Input: part model. Units: mm. Frame: model coordinates. A direction names the side the tool comes from. Give positions to 0.01 mm unless a question says otherwise; leave off trailing zeros. Loops run counter-clockwise (first coordinate to the right, second up) from the corner with the lowest first, then second, coordinate; pieces in that order, holes last. Notation, with made-up numbers: (-17, 84.25) -> (23, 84.25) arc R17 cw to (23, 89.25) -> close; hole circle Ø3 at (-32.5, 34.25). An arc over 180 degrees is marked (long way). Use CSV: the item, a comma, the result in double quotes.
```python
from build123d import *

# Parameters (mm, degrees)
SKETCH1_W                       = 126
SKETCH1_H                       = 106
BOSS_EXTRUDE1_DEPTH             = 5
SKETCH3_W                       = 126
SKETCH3_H                       = 106
SKETCH3_W_2                     = 122
SKETCH3_H_2                     = 102
BOSS_EXTRUDE3_DEPTH             = 5
BOSS_EXTRUDE5_DEPTH             = 4
FILLET1_R                       = 3
F_4_0MM_DOWEL_HOLE1_D           = 4
F_4_0MM_DOWEL_HOLE1_CSINK_D     = 8
F_4_0MM_DOWEL_HOLE1_CSINK_ANGLE = 90
SKETCH17_R                      = 1.15
BOSS_EXTRUDE6_DEPTH             = 10
SKETCH18_W                      = 3
SKETCH18_H                      = 3
BOSS_EXTRUDE7_DEPTH             = 4
SKETCH4_R                       = 3.75
BOSS_EXTRUDE8_DEPTH             = 4
F_2_5MM_DOWEL_HOLE1_D           = 2.5


with BuildPart() as part:
    # Sketch1 → Boss-Extrude1 (new body)
    with BuildSketch(Plane(origin=(0, 0, 0), x_dir=(1, 0, 0), z_dir=(0, 1, 0))):
        Rectangle(SKETCH1_W, SKETCH1_H)
    extrude(amount=BOSS_EXTRUDE1_DEPTH)

    # Sketch3 → Boss-Extrude3 (add)
    with BuildSketch(Plane(origin=(0, 5, 0), x_dir=(1, 0, 0), z_dir=(0, 1, 0))):
        Rectangle(SKETCH3_W, SKETCH3_H)
        Rectangle(SKETCH3_W_2, SKETCH3_H_2, mode=Mode.SUBTRACT)
    extrude(amount=BOSS_EXTRUDE3_DEPTH)

    # Sketch7 → Boss-Extrude5 (add)
    with BuildSketch(Plane(origin=(0, 0, 0), x_dir=(1, 0, 0), z_dir=(0, 1, 0))):
        with BuildLine():
            Line((-63, 43), (-73, 43))
            ThreePointArc((-73, 43), (-78, 38), (-73, 33))
            Line((-73, 33), (-63, 33))
            Line((-63, 33), (-63, 43))
        make_face()
        with BuildLine():
            Line((63, -33), (73, -33))
            ThreePointArc((73, -33), (78, -38), (73, -43))
            Line((73, -43), (63, -43))
            Line((63, -43), (63, -33))
        make_face()
    extrude(amount=BOSS_EXTRUDE5_DEPTH)

    # Fillet1
    fillet1_edges = [part.edges().sort_by_distance(p)[0] for p in [
        (-63, 2, -33),
        (-63, 2, -43),
        (63, 2, 33),
        (63, 2, 43),
    ]]
    fillet(fillet1_edges, radius=FILLET1_R)

    # Ø4.0mm Dowel Hole1 (through all)
    with Locations(Plane(origin=(0, 4, 0), x_dir=(1, 0, 0), z_dir=(0, 1, 0))):
        with Locations((-73, 38), (73, -38)):
            CounterSinkHole(F_4_0MM_DOWEL_HOLE1_D / 2, F_4_0MM_DOWEL_HOLE1_CSINK_D / 2, counter_sink_angle=F_4_0MM_DOWEL_HOLE1_CSINK_ANGLE)

    # Sketch17 → Boss-Extrude6 (add)
    with BuildSketch(Plane(origin=(0, 5, 0), x_dir=(1, 0, 0), z_dir=(0, 1, 0))):
        with Locations(Location((-55.626, -15.47, 0), (0, 0, 90))):
            Circle(SKETCH17_R)
        with Locations(Location((55.626, -15.47, 0), (0, 0, 90))):
            Circle(SKETCH17_R)
    extrude(amount=BOSS_EXTRUDE6_DEPTH)

    # Sketch18 → Boss-Extrude7 (add)
    with BuildSketch(Plane(origin=(0, 5, 0), x_dir=(1, 0, 0), z_dir=(0, 1, 0))):
        with Locations((-59.5, 49.5)):
            Rectangle(SKETCH18_W, SKETCH18_H)
        with Locations((59.5, 49.5)):
            Rectangle(SKETCH18_W, SKETCH18_H)
        with Locations((-59.5, -49.5)):
            Rectangle(SKETCH18_W, SKETCH18_H)
        with Locations((59.5, -49.5)):
            Rectangle(SKETCH18_W, SKETCH18_H)
    extrude(amount=BOSS_EXTRUDE7_DEPTH)

    # Sketch4 → Boss-Extrude8 (add)
    with BuildSketch(Plane(origin=(0, 5, 0), x_dir=(1, 0, 0), z_dir=(0, 1, 0))):
        with Locations(Location((0, 13.486, 0), (0, 0, 90))):
            Circle(SKETCH4_R)
    extrude(amount=BOSS_EXTRUDE8_DEPTH)

    # Ø2.5mm Dowel Hole1 (through all)
    with Locations(Plane(origin=(0, 9, 0), x_dir=(1, 0, 0), z_dir=(0, 1, 0))):
        with Locations((0, 13.486)):
            Hole(F_2_5MM_DOWEL_HOLE1_D / 2)


solid = part.part
```
1) Ray query, line 1 (Z direction, x = -73, y = 0.7); line 2 (Z direction, x = 73, y = 1.4); line 3 (X direction, y = 0.65, z = -38). Return the intervals inside material, ascending.
From the geometry:
line 1,"z = -43 to -40, -36 to -33"
line 2,"z = 33 to 36, 40 to 43"
line 3,"x = -78 to -75, -71 to 63"
2) Section query D-D (z = -28). Return loops of the section in (x, y).
From the geometry:
outline,"(-63, 0) -> (63, 0) -> (63, 10) -> (61, 10) -> (61, 5) -> (-61, 5) -> (-61, 10) -> (-63, 10) -> close"
3) Reachability of faces 1 (the cylindrical face through (-63.86, 2.03, -43.9)), 2 (the flat face through (-60, 7, 48)) from +Z, -Z, +X, -X, +Y, -Y: full face, straight path, thin tool, end or side. Return the list, or none.
From the geometry:
face 1,"-Z, -X, +Y, -Y"
face 2,"+Y"
4) Section query A-A (z = 38). Return loops of the section in (x, y), then the cut area to 3 significant figures.
From the geometry:
outline,"(-63, 0) -> (71, 0) -> (71, 2) -> (69, 4) -> (63, 4) -> (63, 10) -> (61, 10) -> (61, 5) -> (-61, 5) -> (-61, 10) -> (-63, 10) -> close; (75, 0) -> (78, 0) -> (78, 4) -> (77, 4) -> (75, 2) -> close"
area,"690 mm^2"
5) Section query B-B (y = 7.25). Return loops of the section in (x, z), then the cut area to 3 significant figures.
From the geometry:
outline,"(-63, -53) -> (63, -53) -> (63, 53) -> (-63, 53) -> close; circle Ø2.3 at (-55.63, 15.47); circle Ø7.5 at (0, -13.49); circle Ø2.3 at (55.63, 15.47); hole (-61, -48) -> (-58, -48) -> (-58, -51) -> (58, -51) -> (58, -48) -> (61, -48) -> (61, 48) -> (58, 48) -> (58, 51) -> (-58, 51) -> (-58, 48) -> (-61, 48) -> close; hole circle Ø2.5 at (0, -13.49)"
area,"996 mm^2"
6) Contact query for flat-ended pins moving along their axis: pin 1 (4 mm diameter, centred on y = 8, z = -7, fed in from -X); pin 2 (5 mm diameter, centred on x = 61.5, z = 31.5, fed in from +Y); pin 3 (1.5 mm diameter, centred on x = 59, z = 50, fed in from +Y). Output: stop coordinate, or through.
From the geometry:
pin 1,"stops at x = -63"
pin 2,"stops at y = 10"
pin 3,"stops at y = 9"
7) Section query C-C (x = -42). Return loops of the section in (y, z).
From the geometry:
outline,"(0, -53) -> (10, -53) -> (10, -51) -> (5, -51) -> (5, 51) -> (10, 51) -> (10, 53) -> (0, 53) -> close"
8) Mould query, pull axis X, two halves, no side actions, for faces 3 (the cylindrical face through (-78, 2, -38)), 4 (the cylindrical face through (63.86, 2.03, 32.1)), 5 (the flat face through (2, 9, -13)), 6 (the flat face through (-1, 0, -1)). Classes: pulls with the +X half, pulls with the -X half, needs draft (parallel to the pull), parting line crosses it, or undercut.
From the geometry:
face 3,"pulls with the -X half"
face 4,"pulls with the +X half"
face 5,"undercut"
face 6,"needs draft"
